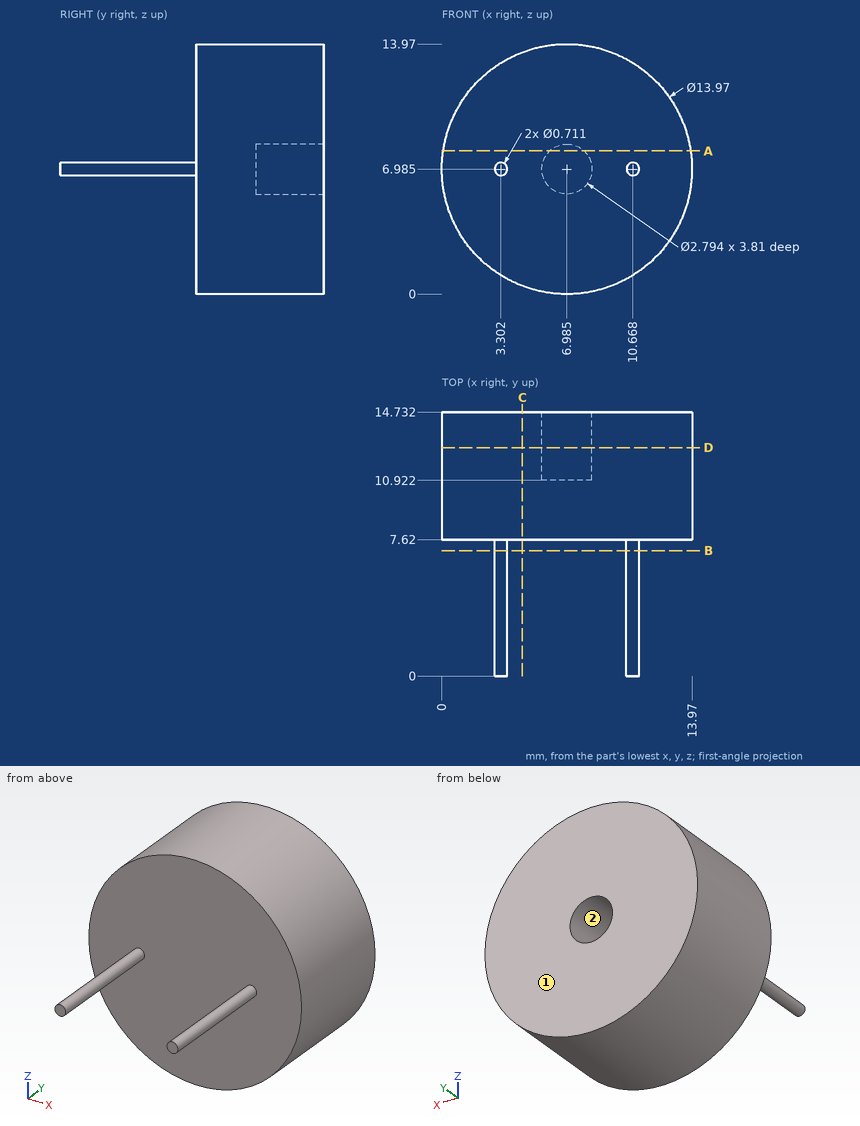
Geometry check sheet. Reference: drawing and pictorial views, mm from the part's lowest x, y, z. A direction names the side the tool comes from. Round coordinates to 2 decimals unless told otherwise and drop trailing zeros. Loops run counter-clockwise (first coordinate to the right, second up) from the corner with the lowest first, then second, coordinate; pieces in that order, holes last. Notation, with made-up numbers: (45.5, -35.75) - (96.5, -35.75) arc R16 cw to (96.5, -20.75) - close; hole circle Ø10 at (72, 32.5). An arc over 180 degrees is marked (long way). Use a Markdown table: item, result. Add a question column.
1. Section check C-C, the plane x = 4.5. Record the boundary of the cut face in (y, z).
2. Section check D-D, the plane y = 12.75. Record the boundary of the cut face in (x, z) (3 decimals), plus the area to 3 significant figures.
3. Section check A-A, the plane z = 8. Record the boundary of the cut face in (x, y) (1 decimal).
4. Thickness scan on probe 1 along X at (y, z) = (2.75, 7); probe 2 along X at (y, z) = (13.5, 7); probe 3 along Y at (x, z) = (5.5, 5). Record the ranges inside material, lowest first. Write a range as [from, to].
5. Section check B-B, the plane y = 7. Record the boundary of the cut face in (x, z) (1 decimal).
6. Gauge pin test, flat ends, axial feed: pin 1 (8 mm diameter, centred on y = 13, z = 9, fed in from -X); pin 2 (1 mm diameter, centred on x = 5, y = 9, fed in from +Z); pin 3 (2 mm diameter, centred on x = 9.5, y = 3, fed in from -Z); pin 4 (2 mm diameter, centred on x = 3, y = 2.5, fed in from +Z). Record the tip position at first contact, or that the pin passes through.
7. Access from +Z, -Z, +X, -X, +Y, -Y to the whole of each face (thin tool, end or side, straight path). Record for the marked faces 1 and 2.
Checks:
| question | item | result |
|---|---|---|
| 1 | outline | (7.62, 0.46) - (14.73, 0.46) - (14.73, 13.51) - (7.62, 13.51) - close |
| 2 | outline | circle Ø13.97 at (6.985, 6.985); hole circle Ø2.794 at (6.985, 6.985) |
| 2 | area | 147 mm^2 |
| 3 | outline | (0.1, 7.6) - (13.9, 7.6) - (13.9, 14.7) - (7.9, 14.7) - (7.9, 10.9) - (6, 10.9) - (6, 14.7) - (0.1, 14.7) - close |
| 4 | probe 1 | x = [2.95, 3.66], [10.31, 11.02] |
| 4 | probe 2 | x = [0, 5.59], [8.38, 13.97] |
| 4 | probe 3 | y = [7.62, 14.73] |
| 5 | outline | circle Ø0.7 at (3.3, 7); circle Ø0.7 at (10.7, 7) |
| 6 | pin 1 | stops at x = 0 |
| 6 | pin 2 | stops at z = 13.81 |
| 6 | pin 3 | stops at z = 6.67 |
| 6 | pin 4 | stops at z = 7.34 |
| 7 | face 1 | +Z, -Z, +X, -X, +Y |
| 7 | face 2 | +Y |
